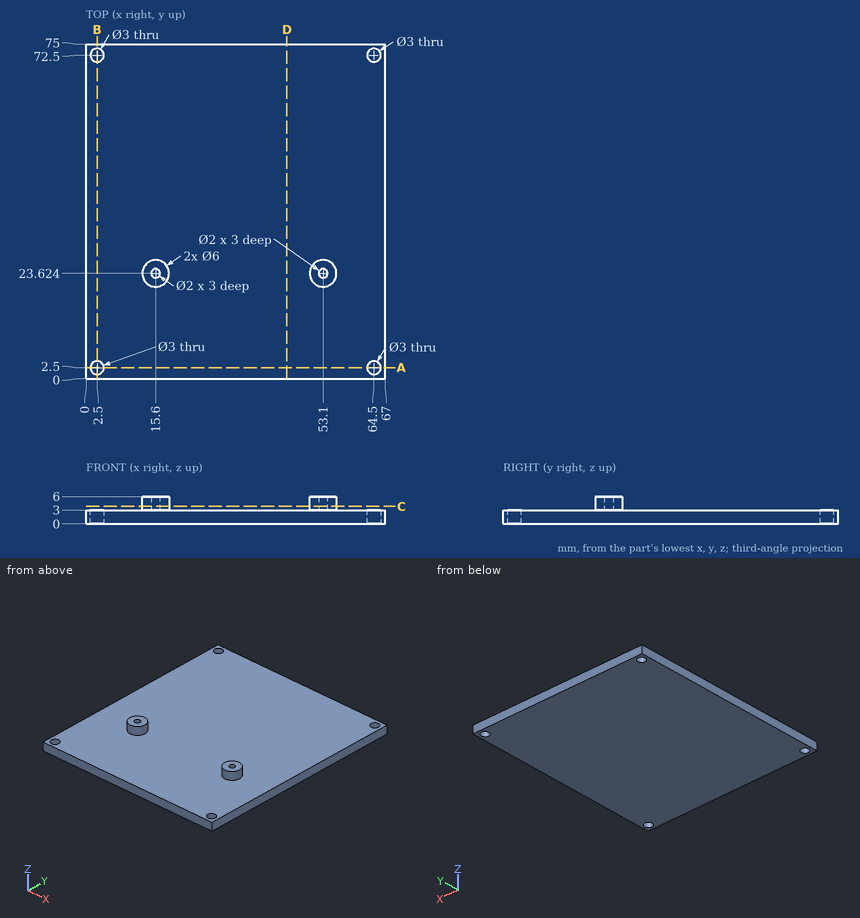
Answer from the drawing. Dimensions are ordinates in mm from the lowest x, y and z of the part. Round coordinates to 2 decimals unless told otherwise and drop trailing zeros. Write each loop counter-clockwise with the first axis right and the second up, starting at its lowest first coordinate (ties: lowest second). Pieces come first, ordered by that corner, then holes. Notation, with made-up numbers: M -32.75,82 L -8.75,82 A20 ccw -8.75,112 Z; hole C 83.25,-17 d3. An arc over 180 degrees is marked long. Write each question's results on one line, items separated by ' | '. Start each with the question number.
Item 1: Straight lines are drawn through the part: probe 1 along Y at (x, z) = (2.5, 1.5); probe 2 along X at (y, z) = (72.5, 1.4); probe 3 along Z at (x, y) = (4.5, 31.5). For each, find the intervals that lie inside material, in ascending order.
Item 2: Find section A-A on y = 2.5. Write down the section's boundary in (x, z).
Item 3: Find section D-D on x = 45. Write down the section's boundary in (y, z).
Item 4: Find section B-B on x = 2.5. Write down the section's boundary in (y, z), and give its area (3 significant figures).
Item 5: Given pin 1 Ø1.2 at (x, y) = (53.1, 23.62) entering from -Z; pin 2 Ø1.6 at (x, y) = (53, 23.5) entering from +Z, each flat-ended and moving along its own axis, determine where each tip first touches the part or whether it passes through.
Item 6: Find section C-C on z = 3.85. Write down the section's boundary in (x, y).
Answer block:
1) probe 1: y = 0 to 1, 4 to 71, 74 to 75 | probe 2: x = 0 to 1, 4 to 63, 66 to 67 | probe 3: z = 0 to 3
2) outline: M 0,0 L 1,0 L 1,3 L 0,3 Z; M 4,0 L 63,0 L 63,3 L 4,3 Z; M 66,0 L 67,0 L 67,3 L 66,3 Z
3) outline: M 0,0 L 75,0 L 75,3 L 0,3 Z
4) outline: M 0,0 L 1,0 L 1,3 L 0,3 Z; M 4,0 L 71,0 L 71,3 L 4,3 Z; M 74,0 L 75,0 L 75,3 L 74,3 Z | area: 207 mm²
5) pin 1: stops at z = 0 | pin 2: stops at z = 3
6) outline: C 15.6,23.62 d6; C 53.1,23.62 d6; hole C 15.6,23.62 d2; hole C 53.1,23.62 d2
